Design review of the part built by this model. Coordinates are the model's own, in mm. A direction names the side the tool comes from. Coordinates: 2 decimals unless noted, no trailing zeros. Loops run counter-clockwise (first coordinate to the right, second up) from the corner with the lowest first, then second, coordinate; pieces in that order, holes last. Notation, with made-up numbers: M 84.5,-22.5 L 132.5,-22.5 A18 cw 132.5,9.5 Z; hole C 60,60.25 d8. An arc over 180 degrees is marked long. Answer as a JSON object with one key per item and string values. Group by question number.
1. Draft analysis for pull direction Z (two halves, no side actions). For faces 4 (the cylindrical face through (-1.479, -18.871, -27.546)), 5 (the cylindrical face through (7.4, 11.87, -27.21)), 6 (the flat face through (7, 23.977, 17)), state which applies: +Z half, -Z half, draft (parallel to the pull), parting line (faces both ways), or undercut.
2. Machinability: for faces 1 (the cylindrical face through (7.4, 1.51, -13.07)), 2 (the cylindrical face through (7.395, 9.723, 52.04)), 3 (the flat face through (7, -0.062, 16)), which of the approach directions +Z, -Z, +X, -X, +Y, -Y give a long, thin tool a straight path to every point of the face, cutting with its end or side? Answer none if there is none.
3. Consider section C-C (x = 1.25). State the section outline as (y, z) points.
4. To check wall thickness, follow probe 1 along X at (y, z) = (-6.5, -6.5); probe 2 along Z at (x, y) = (4.25, 11.5); probe 3 along Y at (x, z) = (8.75, -2). State the ranges of each line that lie inside material, in increasing order.
5. Consider section D-D (y = 8.5). State the section outline as (x, z) points, then the cut area to 3 significant figures.
6. Insertion check: pin 1 (7.5 mm diameter, centred on x = 7, z = 14, fed in from -Y). The pin has a flat end and moves straight along its axis. Give the tip position at first contact, or say it passes through.
7. Consider section B-B (z = 2.5). State the section outline as (x, y) points.
8. Consider section A-A (y = -11.5). State the section outline as (x, z) points, then the cut area to 3 significant figures.
from build123d import *

# Parameters (mm, degrees)
RESSALTO_EXTRUS_O2_DEPTH = 15
RESSALTO_EXTRUS_O3_DEPTH = 3
RESSALTO_EXTRUS_O4_DEPTH = 3


with BuildPart() as part:
    # Esboço2 → Ressalto-extrusão2 (new body)
    with BuildSketch(Plane(origin=(0, 0, 0), x_dir=(0, 0, -1), z_dir=(1, 0, 0))):
        with BuildLine():
            Line((2.90159992, -0.062465938), (-35.09840008, -0.062465938))
            Line((-35.09840008, -0.062465938), (-39.886084903, -0.062465938))
            ThreePointArc((-39.886084903, -0.062465938), (-45.202180234, 1.467638524), (-48.891439328, 5.589707975))
            ThreePointArc((-48.891439328, 5.589707975), (-52.096536948, 9.772081499), (-56.69840008, 12.338743681))
            ThreePointArc((-56.69840008, 12.338743681), (-59.373224015, 11.895603401), (-60.59840008, 9.476926077))
            Line((-60.59840008, 9.476926077), (-60.59840008, 20.976926077))
            ThreePointArc((-60.59840008, 20.976926077), (-59.719720424, 23.09824642), (-57.59840008, 23.976926077))
            Line((-57.59840008, 23.976926077), (25.40159992, 23.976926077))
            ThreePointArc((25.40159992, 23.976926077), (27.522920263, 23.09824642), (28.40159992, 20.976926077))
            Line((28.40159992, 20.976926077), (28.40159992, 9.476926077))
            ThreePointArc((28.40159992, 9.476926077), (27.176423855, 11.895603401), (24.50159992, 12.338743681))
            ThreePointArc((24.50159992, 12.338743681), (19.899736788, 9.772081499), (16.694639168, 5.589707975))
            ThreePointArc((16.694639168, 5.589707975), (13.005380073, 1.467638524), (7.689284743, -0.062465938))
            Line((7.689284743, -0.062465938), (2.90159992, -0.062465938))
        make_face()
    extrude(amount=RESSALTO_EXTRUS_O2_DEPTH)

    # Esboço3 → Ressalto-extrusão3 (add)
    with BuildSketch(Plane.ZY):
        with BuildLine():
            Line((60.59840008, 15.226926077), (60.59840008, 20.976926077))
            ThreePointArc((60.59840008, 20.976926077), (59.719720424, 23.09824642), (57.59840008, 23.976926077))
            Line((57.59840008, 23.976926077), (16.09840008, 23.976926077))
            Line((16.09840008, 23.976926077), (-25.40159992, 23.976926077))
            ThreePointArc((-25.40159992, 23.976926077), (-27.522920263, 23.09824642), (-28.40159992, 20.976926077))
            Line((-28.40159992, 20.976926077), (-28.40159992, 15.226926077))
            Line((-28.40159992, 15.226926077), (-28.40159992, -16.773073923))
            ThreePointArc((-28.40159992, -16.773073923), (-27.522920263, -18.894394267), (-25.40159992, -19.773073923))
            Line((-25.40159992, -19.773073923), (57.59840008, -19.773073923))
            ThreePointArc((57.59840008, -19.773073923), (59.719720424, -18.894394267), (60.59840008, -16.773073923))
            Line((60.59840008, -16.773073923), (60.59840008, 15.226926077))
        make_face()
    extrude(amount=RESSALTO_EXTRUS_O3_DEPTH)

    # Esboço4 → Ressalto-extrusão4 (add)
    with BuildSketch(Plane(origin=(15, 0, 0), x_dir=(0, 0, -1), z_dir=(1, 0, 0))):
        with BuildLine():
            Line((-16.09840008, 23.976926077), (25.40159992, 23.976926077))
            ThreePointArc((25.40159992, 23.976926077), (27.522920263, 23.09824642), (28.40159992, 20.976926077))
            Line((28.40159992, 20.976926077), (28.40159992, 15.226926077))
            Line((28.40159992, 15.226926077), (28.40159992, -16.773073923))
            ThreePointArc((28.40159992, -16.773073923), (27.522920263, -18.894394267), (25.40159992, -19.773073923))
            Line((25.40159992, -19.773073923), (-57.59840008, -19.773073923))
            ThreePointArc((-57.59840008, -19.773073923), (-59.719720424, -18.894394267), (-60.59840008, -16.773073923))
            Line((-60.59840008, -16.773073923), (-60.59840008, 15.226926077))
            Line((-60.59840008, 15.226926077), (-60.59840008, 20.976926077))
            ThreePointArc((-60.59840008, 20.976926077), (-59.719720424, 23.09824642), (-57.59840008, 23.976926077))
            Line((-57.59840008, 23.976926077), (-16.09840008, 23.976926077))
        make_face()
    extrude(amount=RESSALTO_EXTRUS_O4_DEPTH)


solid = part.part
Findings below:
{
 "1": {"face 4": "-Z half", "face 5": "undercut", "face 6": "draft"},
 "2": {"face 1": "-Z, -Y", "face 2": "-Y", "face 3": "+Z, -Z, -Y"},
 "3": {"outline": "M -0.06,-7.69 A10 ccw 5.59,-16.69 A13 cw 12.34,-24.5 A3 cw 9.48,-28.4 L 20.98,-28.4 A3 ccw 23.98,-25.4 L 23.98,57.6 A3 ccw 20.98,60.6 L 9.48,60.6 A3 cw 12.34,56.7 A13 cw 5.59,48.89 A10 ccw -0.06,39.89 Z"},
 "4": {"probe 1": "x = -3 to 0, 15 to 18", "probe 2": "z = -28.4 to -27.62, -22.46 to 54.66, 59.81 to 60.6", "probe 3": "y = -0.06 to 23.98"},
 "5": {"outline": "M -3,-28.4 L 0,-28.4 L 0,-18.62 L 15,-18.62 L 15,-28.4 L 18,-28.4 L 18,60.6 L 15,60.6 L 15,50.82 L 0,50.82 L 0,60.6 L -3,60.6 Z", "area": "1,580 mm^2"},
 "6": {"pin 1": "stops at y = -0.06"},
 "7": {"outline": "M -3,-19.77 L 0,-19.77 L 0,-0.06 L 15,-0.06 L 15,-19.77 L 18,-19.77 L 18,23.98 L -3,23.98 Z"},
 "8": {"outline": "M -3,-28.4 L 0,-28.4 L 0,60.6 L -3,60.6 Z; M 15,-28.4 L 18,-28.4 L 18,60.6 L 15,60.6 Z", "area": "534 mm^2"}
}
